```python
from build123d import *

# Parameters (mm, degrees)
F0_W     = 16
F0_H     = 5
F1_DEPTH = 28
F2_W     = 52
F2_H     = 49.263156
F3_DEPTH = 74.4
F4_R     = 5
F5_R     = 2.5
F6_DEPTH = 3.301


with BuildPart() as f1:
    # F0 (on Right) → F1 (new body, symmetric)
    with BuildSketch(Plane.YZ):
        with BuildLine():
            Line((-14, 75.869719), (-14, 0))
            Line((-14, 0), (14, 0))
            Line((14, 0), (14, 75.869719))
            ThreePointArc((14, 75.869719), (13.463923, 77.163923), (12.169719, 77.7))
            Line((12.169719, 77.7), (5, 77.7))
            ThreePointArc((5, 77.7), (0, 72.7), (-5, 77.7))
            Line((-5, 77.7), (-12.169719, 77.7))
            ThreePointArc((-12.169719, 77.7), (-13.463923, 77.163923), (-14, 75.869719))
        make_face()
        with Locations((0, 15.5)):
            Rectangle(F0_W, F0_H, mode=Mode.SUBTRACT)
        with Locations((0, 25.5)):
            Rectangle(F0_W, F0_H, mode=Mode.SUBTRACT)
        with Locations((0, 35.5)):
            Rectangle(F0_W, F0_H, mode=Mode.SUBTRACT)
        with Locations((0, 45.5)):
            Rectangle(F0_W, F0_H, mode=Mode.SUBTRACT)
        with Locations((0, 55.5)):
            Rectangle(F0_W, F0_H, mode=Mode.SUBTRACT)
    extrude(amount=F1_DEPTH, both=True)

    # F2 (on face) → F3 (cut)
    with BuildSketch(Plane.XY.offset(77.7)):
        with Locations((0, 0.389209)):
            Rectangle(F2_W, F2_H)
    extrude(amount=-F3_DEPTH, mode=Mode.SUBTRACT)

    # F4
    f4_edges = [f1.edges().sort_by_distance(p)[0] for p in [
        (-28, 0, 0),
        (28, 0, 0),
        (-26, 0, 3.3),
        (26, 0, 3.3),
    ]]
    fillet(f4_edges, radius=F4_R)

    # F5 (on face) → F6 (cut, through all)
    with BuildSketch(Plane.XY.offset(3.3)):
        Circle(F5_R)
    extrude(amount=-F6_DEPTH, mode=Mode.SUBTRACT)


solid = f1.part
```
CAD build for the part. Positions are in the model's coordinates, mm. A direction names the side the tool comes from. Round coordinates to 2 decimals unless told otherwise and drop trailing zeros. Write each loop counter-clockwise with the first axis right and the second up, starting at its lowest first coordinate (ties: lowest second). Pieces come first, ordered by that corner, then holes.
Item 1: Band-saw the part on C-C on y = -10.25. Write the cut outline in (x, z).
Filled in:
outline: (-28, 5) arc R5 ccw to (-23, 0) - (23, 0) arc R5 ccw to (28, 5) - (28, 77.7) - (26, 77.7) - (26, 8.3) arc R5 cw to (21, 3.3) - (-21, 3.3) arc R5 cw to (-26, 8.3) - (-26, 77.7) - (-28, 77.7) - close
Item 2: Mould opens along Y. For faces 4 (the flat face through (27, 8, 35)), 5 (the cylindrical face through (27.01, 13.48, 77.15)), 6 (the flat face through (-27, 9, 77.7)) say: released by +Y, released by -Y, zero draft, split by the parting line, or undercut.
Filled in:
face 4: undercut
face 5: released by +Y
face 6: zero draft
Item 3: Drop flat-ended pins along their axis: pin 1 Ø1.6 at (x, y) = (27, -3.5) entering from +Z; pin 2 Ø8 at (x, y) = (-21.5, -8) entering from +Z; pin 3 Ø1.5 at (x, y) = (-10, 2) entering from +Z. Give the stop position or say it passes through.
Filled in:
pin 1: stops at z = 75.15
pin 2: stops at z = 6.12
pin 3: stops at z = 3.3
Item 4: Drill centre lines: L1, parallel to X at y = -12.25, z = 56; L2, parallel to Z at x = 7.5, y = 0.5; L3, parallel to Y at x = 0, z = 2.35. Where is each one in solid material? Low to high.
Filled in:
L1: x = -28 to -26, 26 to 28
L2: z = 0 to 3.3
L3: y = -14 to -2.5, 2.5 to 14
Item 5: Band-saw the part on D-D on y = 0. Give the number of separate pieces and of enclosed holes in the cut face, then the cut area to 3 significant figures.
Filled in:
separate pieces: 12
enclosed holes: 0
area: 346 mm2
Item 6: Band-saw the part on A-A on z = 19. Write the cut outline in (x, y), then the cut area to 3 significant figures.
Filled in:
outline: (-28, -14) - (-26, -14) - (-26, 14) - (-28, 14) - close; (26, -14) - (28, -14) - (28, 14) - (26, 14) - close
area: 112 mm2
Item 7: Band-saw the part on B-B on x = 0. Write the cut outline in (y, z), then the cut area to 3 significant figures.
Filled in:
outline: (-14, 0) - (-2.5, 0) - (-2.5, 3.3) - (-14, 3.3) - close; (2.5, 0) - (14, 0) - (14, 3.3) - (2.5, 3.3) - close
area: 75.9 mm2
Item 8: Tool access for faces 1 (the flat face through (0, 3, 3.3)), 2 (the flat face through (28, 0, 42)), 3 (the flat face through (27, 0, 23)): list every direction of +Z, -Z, +X, -X, +Y, -Y with a clear straight run to the whole face (end or side of a thin tool).
Filled in:
face 1: +Z, +Y, -Y
face 2: +Z, -Z, +X, +Y, -Y
face 3: +X, -X
